Autodesk Inventor part; units mm, degrees
ref_plane "YZ Plane" through (0, 0, 0) normal (1, 0, 0) x (0, 1, 0)
ref_plane "XZ Plane" through (0, 0, 0) normal (0, 1, 0) x (-1, 0, 0)
ref_plane "XY Plane" through (0, 0, 0) normal (0, 0, 1) x (1, 0, 0)
sketch "Sketch1" plane through (0, 0, 0) normal (0, 1, 0) x (-1, 0, 0)
  line L0 (100.7745, 123.6) -> (-100.7745, 123.6)
  line L1 (-100.7745, 123.6) -> (-100.7745, -123.6)
  line L2 (-100.7745, -123.6) -> (100.7745, -123.6)
  line L3 (100.7745, -123.6) -> (100.7745, 123.6)
  point P0 (0, 0)
  point P1 (100.7745, 0)
  point P2 (0, 123.6)
  dimension "d0" = 247.2
  dimension "d1" = 201.549
extrude "Extrusion1" add sketch "Sketch1" along normal blind 56.4
sketch "Sketch3" plane through (100.7745, 0, 123.6) normal (1, 0, 0) x (0, 0, -1)
  circle A0 centre (30.111, 15.25) radius 11.25
  circle A1 centre (217.089, 15.25) radius 11.25
  line L0 (247.2, 0) -> (0, 0)
  line L1 (0, 0) -> (0, 56.4)
  line L2 (247.2, 56.4) -> (0, 56.4)
  line L3 (247.2, 0) -> (247.2, 56.4)
  point P0 (123.6, 0)
  dimension "d12" = 4
  dimension "d13" = 4
  dimension "d50" = 30.111
  dimension "d51" = 15.25
  dimension "d52" = 15.25
  dimension "d53" = 30.111
extrude "Extrusion3" add sketch "Sketch3" along normal blind 30.94 contours A0 | A1
sketch "Sketch5" plane through (-100.7745, 0, -123.6) normal (-1, 0, 0) x (0, 0, 1)
  circle A0 centre (217.089, 15.25) radius 11.25
  circle A1 centre (30.111, 15.25) radius 11.25
  circle A2 centre (30.111, 15.25) radius 11.25
  circle A3 centre (217.089, 15.25) radius 11.25
  point P0 (123.6, 0)
extrude "Extrusion5" add sketch "Sketch5" along normal blind 30.94
sketch "Sketch8" plane through (100.7745, 0, 123.6) normal (1, 0, 0) x (0, 0, -1)
  line L0 (0, 0) -> (0, 56.4)
  line L1 (0, 47.0005) -> (9.3472, 56.4)
  line L2 (0, 9.3995) -> (9.3472, 0)
  line L3 (0, 56.4) -> (247.2, 56.4)
  line L4 (237.8528, 56.4) -> (247.2, 47.0005)
  line L5 (247.2, 0) -> (247.2, 56.4)
  line L6 (247.2, 9.3995) -> (237.8528, 0)
  line L7 (0, 0) -> (247.2, 0)
  point P0 (123.6, 0)
  dimension "d22" = 13.256
  dimension "d23" = 135.16
  dimension "d24" = 135.16
  dimension "d25" = 135.16
  dimension "d26" = 135.16
extrude "Extrusion6" cut sketch "Sketch8" against normal through all contours L0 L2 L7 | L0 L3 L1 | L6 L5 L7 | L3 L5 L4
sketch "Sketch9" plane through (0, 56.4, 0) normal (0, 1, 0) x (1, 0, 0)
  circle A0 centre (78.9745, -93.586) radius 1.651
  line L0 (100.7745, -123.6) -> (-100.7745, -123.6)
  line L1 (100.7745, -114.2528) -> (100.7745, 114.2528)
  circle A1 centre (78.9745, 93.586) radius 1.651
  circle A2 centre (-78.9745, 93.586) radius 1.651
  circle A3 centre (-78.9745, -93.586) radius 1.651
  line L2 (-100.7745, 123.6) -> (100.7745, 123.6)
  line L3 (-100.7745, 114.2528) -> (-100.7745, -114.2528)
  point P0 (0, 0)
  dimension "d29" = 30.014
  dimension "d30" = 21.8
  dimension "d31" = 3.302
  dimension "d32" = 3.302
  dimension "d33" = 3.302
  dimension "d34" = 3.302
  dimension "d35" = 21.8
  dimension "d36" = 30.014
  dimension "d37" = 21.8
  dimension "d38" = 30.014
  dimension "d39" = 21.8
  dimension "d40" = 30.014
extrude "Extrusion7" add sketch "Sketch9" along normal blind 4.763
sketch "Sketch10" plane through (0, 56.4, 0) normal (0, 1, 0) x (1, 0, 0)
  circle A0 centre (76.4345, 63.106) radius 1.905
  circle A1 centre (76.4345, 6.591) radius 1.905
  line L0 (100.7745, -114.2528) -> (100.7745, 114.2528)
  line L1 (-100.7745, 123.6) -> (100.7745, 123.6)
  point P0 (0, 0)
  dimension "d43" = 24.34
  dimension "d44" = 3.81
  dimension "d45" = 3.81
  dimension "d46" = 60.494
  dimension "d47" = 56.515
extrude "Extrusion8" add sketch "Sketch10" along normal blind 6.35
fillet "Fillet1" radius 2 4 edges at (131.7145, 15.25, 104.739) (131.7145, 15.25, -82.239) (-131.7145, 15.25, -104.739) (-131.7145, 15.25, 82.239)
sketch "Sketch11" plane through (0, 56.4, 0) normal (0, 1, 0) x (1, 0, 0)
  circle A0 centre (76.4345, 63.106) radius 1.905
  circle A1 centre (76.4345, 6.591) radius 1.905
  circle A2 centre (-78.9745, 93.586) radius 1.651
  circle A3 centre (78.9745, -93.586) radius 1.651
  circle A4 centre (78.9745, 93.586) radius 1.651
  circle A5 centre (-78.9745, -93.586) radius 1.651
  line L0 (100.7745, 114.2528) -> (-100.7745, 114.2528)
  line L1 (-100.7745, 114.2528) -> (-100.7745, -114.2528)
  line L2 (-100.7745, -114.2528) -> (100.7745, -114.2528)
  line L3 (100.7745, -114.2528) -> (100.7745, 114.2528)
  circle A6 centre (-43.9615, 56.5758) radius 1.651
  circle A7 centre (-52.8515, 92.6438) radius 1.651
  circle A8 centre (52.8815, 92.6438) radius 1.651
  circle A9 centre (43.9915, 56.5758) radius 1.651
  point P0 (0, 0)
  dimension "d58" = 21.609
  dimension "d62" = 21.609
  dimension "d63" = 3.302
  dimension "d79" = 87.953
  dimension "d80" = 105.733
  dimension "d81" = 36.068
  dimension "d82" = 36.068
  dimension "d83" = 47.893
  dimension "d84" = 56.783
extrude "Extrusion9" add sketch "Sketch11" along normal blind 6.35 contours A6 | A7 | A8 | A9
sketch "Sketch12" plane through (0, 56.4, 0) normal (0, 1, 0) x (1, 0, 0)
  circle A0 centre (52.8815, 92.6438) radius 1.651
  circle A1 centre (-43.9615, 56.5758) radius 1.651
  circle A2 centre (-52.8515, 92.6438) radius 1.651
  circle A3 centre (43.9915, 56.5758) radius 1.651
  circle A4 centre (76.4345, 63.106) radius 1.905
  circle A5 centre (76.4345, 6.591) radius 1.905
  circle A6 centre (-78.9745, 93.586) radius 1.651
  circle A7 centre (78.9745, -93.586) radius 1.651
  circle A8 centre (78.9745, 93.586) radius 1.651
  circle A9 centre (-78.9745, -93.586) radius 1.651
  line L0 (100.7745, 114.2528) -> (-100.7745, 114.2528)
  line L1 (-100.7745, 114.2528) -> (-100.7745, -114.2528)
  line L2 (-100.7745, -114.2528) -> (100.7745, -114.2528)
  line L3 (100.7745, -114.2528) -> (100.7745, 114.2528)
  circle A10 centre (-72.8345, 20.3292) radius 2.9845
  circle A11 centre (17.0815, 20.3292) radius 2.9845
  circle A12 centre (17.0815, -74.1588) radius 2.9845
  circle A13 centre (-72.8345, -74.1588) radius 2.9845
  point P0 (0, 0)
  dimension "d66" = 27.94
  dimension "d67" = 27.94
  dimension "d68" = 117.856
  dimension "d69" = 117.856
  dimension "d70" = 40.094
  dimension "d71" = 40.094
  dimension "d74" = 5.969
  dimension "d77" = 94.488
  dimension "d78" = 94.488
extrude "Extrusion10" add sketch "Sketch12" along normal blind 34.922 contours A10 | A11 | A12 | A13
equation "\"d13\" = d12"
equation "\"d52\" = d51"
equation "\"d53\" = d50"
equation "\"d24\" = d23"
equation "\"d25\" = d23"
equation "\"d26\" = d23"
equation "\"d32\" = d31"
equation "\"d33\" = d31"
equation "\"d34\" = d31"
equation "\"d35\" = d30"
equation "\"d36\" = d29"
equation "\"d37\" = d30"
equation "\"d38\" = d29"
equation "\"d39\" = d30"
equation "\"d40\" = d29"
equation "\"d45\" = d44"
equation "\"d62\" = d58"
equation "\"d82\" = d81"
equation "\"d67\" = d66"
equation "\"d69\" = d68"
equation "\"d71\" = d70"
equation "\"d78\" = d77"
properties part number "chassis"
Design review of the part built by this model. Coordinates are the model's own, in mm. A direction names the side the tool comes from. Coordinates: 2 decimals unless noted, no trailing zeros. Loops run counter-clockwise (first coordinate to the right, second up) from the corner with the lowest first, then second, coordinate; pieces in that order, holes last. Notation, with made-up numbers: (86.5, 83) -> (108.5, 83) arc R14 cw to (108.5, 89) -> close; hole circle Ø8 at (-18, 87). An arc over 180 degrees is marked (long way). Use a Markdown table: item, result. Add a question column.
Item 1: We need section B-B, the plane y = 15.25. Write out the cut boundary in (x, z).
Item 2: Clearance check with flat-ended pins moving along their axes: P1, Ø2.5, axis at x = -78.5, z = -94, coming from the +Y side; P2, Ø12, axis at y = 42, z = 48, coming from the +X side; P3, Ø5, axis at x = -18, z = 55, coming from the +Y side. State where each tip first meets the part, or that it passes through.
Item 3: Wall thickness on L1, parallel to X at y = 38, z = -3.5; L2, parallel to Y at x = -7.5, z = 2; L3, parallel to X at y = 87, z = 72: over which ranges is each line inside the solid? List them lowest first. Write a range as from..to.
Item 4: We need section A-A, the plane x = 97.5. Write out the cut boundary in (y, z), and give its area (3 significant figures).
Item 5: We need section C-C, the plane z = 46. Write out the cut boundary in (x, y).
Item 6: We need section D-D, the plane y = 43. Write out the cut boundary in (x, z).
Item 7: Machinability: for faces 1 (the cylindrical face through (-69.99, 73.62, 75.06)), 2 (the flat face through (1.411, 51.766, -118.861)), 3 (the cylindrical face through (-115.04, 19.56, 103.88)), which of the approach directions +Z, -Z, +X, -X, +Y, -Y give a long, thin tool a straight path to every point of the face, cutting with its end or side? Answer none if there is none.
Item 8: The part is to be moulded in two halves that separate along X. For faces 4 (the cylindrical face through (115.04, 19.56, -103.88)), 5 (the flat face through (131.714, 15, -93)), 6 (the cylindrical face through (-70.078, 73.617, -21.472)), say which applies: +X half, -X half, draft (parallel to the pull), parting line (faces both ways), or undercut.
Numbers:
| question | item | result |
|---|---|---|
| 1 | outline | (-131.71, -102.74) arc R2 ccw to (-129.71, -104.74) -> (-100.77, -104.74) -> (-100.77, -123.6) -> (100.77, -123.6) -> (100.77, -104.74) -> (129.71, -104.74) arc R2 ccw to (131.71, -102.74) -> (131.71, -84.24) arc R2 ccw to (129.71, -82.24) -> (100.77, -82.24) -> (100.77, 82.24) -> (129.71, 82.24) arc R2 ccw to (131.71, 84.24) -> (131.71, 102.74) arc R2 ccw to (129.71, 104.74) -> (100.77, 104.74) -> (100.77, 123.6) -> (-100.77, 123.6) -> (-100.77, 104.74) -> (-129.71, 104.74) arc R2 ccw to (-131.71, 102.74) -> (-131.71, 84.24) arc R2 ccw to (-129.71, 82.24) -> (-100.77, 82.24) -> (-100.77, -82.24) -> (-129.71, -82.24) arc R2 ccw to (-131.71, -84.24) -> close |
| 2 | P1 | stops at y = 61.16 |
| 2 | P2 | stops at x = 100.77 |
| 2 | P3 | stops at y = 56.4 |
| 3 | L1 | x = -100.77..100.77 |
| 3 | L2 | y = 0..56.4 |
| 3 | L3 | x = -74.9..-70.77, 15.02..19.14 |
| 4 | outline | (0, -114.25) -> (9.4, -123.6) -> (47, -123.6) -> (56.4, -114.25) -> (56.4, 114.25) -> (47, 123.6) -> (9.4, 123.6) -> (0, 114.25) -> close |
| 4 | area | 13,800 mm^2 |
| 5 | outline | (-100.77, 0) -> (100.77, 0) -> (100.77, 56.4) -> (-100.77, 56.4) -> close |
| 6 | outline | (-100.77, -123.6) -> (100.77, -123.6) -> (100.77, 123.6) -> (-100.77, 123.6) -> close |
| 7 | face 1 | +Y |
| 7 | face 2 | -Z, +X, -X, +Y |
| 7 | face 3 | -X |
| 8 | face 4 | draft |
| 8 | face 5 | +X half |
| 8 | face 6 | undercut |
